Verification items for the finished model (mm, model axes). A direction names the side the tool comes from. Round coordinates to 2 decimals unless told otherwise and drop trailing zeros. Write each loop counter-clockwise with the first axis right and the second up, starting at its lowest first coordinate (ties: lowest second). Pieces come first, ordered by that corner, then holes. Notation, with made-up numbers: M 81,83.5 L 92,83.5 A12 cw 92,103.5 Z; hole C -14,48.25 d7. An arc over 180 degrees is marked long. One line per item, written item: value. Start each with the question number.
Item 1: Section check D-D, the plane y = -5.25. Record the cut outline in (x, z), then the cut area to 3 significant figures.
Item 2: Section check A-A, the plane y = -0.5. Record the cut outline in (x, z), then the cut area to 3 significant figures.
Item 3: Gauge pin test, flat ends, axial feed: pin 1 (6 mm diameter, centred on x = -5, y = -3, fed in from -Z); pin 2 (6.5 mm diameter, centred on x = 0, y = 0, fed in from +Z); pin 3 (1 mm diameter, centred on x = -5, z = 3.5, fed in from +Y); pin 4 (1.5 mm diameter, centred on x = -1.5, z = 1.5, fed in from -Y). Record the tip position at first contact, or that the pin passes through.
Item 4: Thickness scan on probe 1 along Z at (x, y) = (7.25, -0.75); probe 2 along Y at (x, z) = (0, 2.5); probe 3 along X at (y, z) = (1.5, 5). Record the ranges inside material, lowest first. Write a range as from..to.
Item 5: Section check B-B, the plane z = 2.75. Record the cut outline in (x, y).
Item 6: Tool access check on faces 4 (the face through (3.222, -5.062, 4.465)), 5 (the face through (-3.222, 5.062, 4.465)), 6 (the face through (-3, 5.4, 2)), 7 (the face through (2.773, 5.321, 4.465)), 8 (the face through (-5.995, -0.259, 4.465)). Record the directions out of +Z, -Z, +X, -X, +Y, -Y that give a thin tool (end or side, any length) a straight path to the whole face; none if there is none.
Item 7: Draft check along X on faces 1 (the face through (5.995, 0.259, 4.465)), 2 (the face through (3.233, -1.341, 3.549)), 3 (the face through (-2.773, -5.321, 4.465)). Enter one of: +X half, -X half, draft (parallel to the pull), parting line (faces both ways), or undercut.
Item 8: Section check C-C, the plane x = 0. Record the cut outline in (y, z), then the cut area to 3 significant figures.
from build123d import *

# Parameters (mm, degrees)
F0_R     = 8
F1_DEPTH = 2
F3_DEPTH = 5
F4_R     = 3.5
F5_DEPTH = 25


with BuildPart() as f1:
    # F0 (on Top) → F1 (new body)
    with BuildSketch(Plane.XY):
        Circle(F0_R)
    extrude(amount=F1_DEPTH)

    # F2 (on face) → F3 (join)
    with BuildSketch(Plane.XY.offset(2)):
        Polygon((5.814557, 3.767084), (-0.355112, 6.919096), (-6.169669, 3.152012), (-5.814557, -3.767084), (0.355112, -6.919096), (6.169669, -3.152012), align=None)
    extrude(amount=F3_DEPTH)

    # F4 (on face) → F5 (cut)
    with BuildSketch(Plane.XY.offset(7)):
        Circle(F4_R)
    extrude(amount=-F5_DEPTH, mode=Mode.SUBTRACT)


solid = f1.part
Response values:
1. outline: M -6.04,0 L 6.04,0 L 6.04,2 L 2.93,2 L 2.93,7 L -2.91,7 L -2.91,2 L -6.04,2 Z
1. area: 53.4 mm2
2. outline: M -7.98,0 L -3.46,0 L -3.46,7 L -5.98,7 L -5.98,2 L -7.98,2 Z; M 3.46,0 L 7.98,0 L 7.98,2 L 6.03,2 L 6.03,7 L 3.46,7 Z
2. area: 43.5 mm2
3. pin 1: stops at z = 0
3. pin 2: passes through
3. pin 3: stops at y = 4.23
3. pin 4: stops at y = -7.96
4. probe 1: z = 0..2
4. probe 2: y = -6.74..-3.5, 3.5..6.74
4. probe 3: x = -6.08..-3.16, 3.16..5.93
5. outline: M -6.17,3.15 L -5.81,-3.77 L 0.36,-6.92 L 6.17,-3.15 L 5.81,3.77 L -0.36,6.92 Z; hole C 0,0 d7
6. face 4: +Z, +X, -Y
6. face 5: +Z, -X, +Y
6. face 6: +Z
6. face 7: +Z, +X, +Y
6. face 8: +Z, -X, -Y
7. face 1: +X half
7. face 2: undercut
7. face 3: -X half
8. outline: M -8,0 L -3.5,0 L -3.5,7 L -6.74,7 L -6.74,2 L -8,2 Z; M 3.5,0 L 8,0 L 8,2 L 6.74,2 L 6.74,7 L 3.5,7 Z
8. area: 50.4 mm2
